Design review of the part built by this model. Coordinates are the model's own, in mm. Give positions to 0.01 mm unless a question says otherwise; leave off trailing zeros. Order: outer loops, then holes, each group sorted by start corner. A loop starts at its lowest first (then second) coordinate and runs counter-clockwise, first axis right, second up. Notation, with made-up numbers: M 78.25,-33.75 L 136.25,-33.75 A32 cw 136.25,5.25 Z; hole C 13.5,44.5 d2. An arc over 180 degrees is marked long. Answer as a JSON object with one key per item and string values.
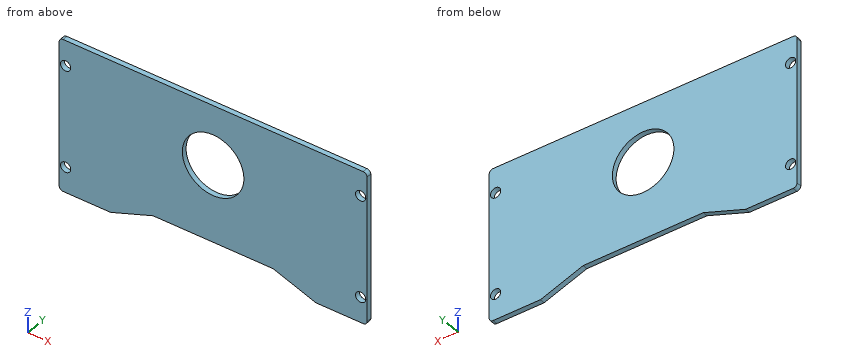
from build123d import *

# Parameters (mm, degrees)
SKETCH_1_W          = 120
SKETCH_1_H          = 60
EXTRUDE_1_DEPTH     = 2
SKETCH_2_R          = 2
CUT_EXTRUDE_1_DEPTH = 2
SKETCH_3_R          = 12
CUT_EXTRUDE_2_DEPTH = 2
FILLET_1_R          = 1.5


with BuildPart() as part:
    # 草图1 → 凸台-拉伸1 (new body)
    with BuildSketch(Plane(origin=(0, 0, 0), x_dir=(1, 0, 0), z_dir=(0, 1, 0))):
        with Locations((60, 30)):
            Rectangle(SKETCH_1_W, SKETCH_1_H)
    extrude(amount=EXTRUDE_1_DEPTH)

    # 草图2 → 切除-拉伸1 (cut)
    with BuildSketch(Plane(origin=(0, 2, 0), x_dir=(1, 0, 0), z_dir=(0, 1, 0))):
        with Locations(Location((117.5, 50, 0), (0, 0, 270))):
            Circle(SKETCH_2_R)
        with Locations(Location((117.5, 10, 0), (0, 0, 90))):
            Circle(SKETCH_2_R)
        with Locations(Location((2.5, 50, 0), (0, 0, 90))):
            Circle(SKETCH_2_R)
        with Locations(Location((2.5, 10, 0), (0, 0, 270))):
            Circle(SKETCH_2_R)
    extrude(amount=-CUT_EXTRUDE_1_DEPTH, mode=Mode.SUBTRACT)

    # 草图3 → 切除-拉伸2 (cut)
    with BuildSketch(Plane(origin=(0, 2, 0), x_dir=(1, 0, 0), z_dir=(0, 1, 0))):
        with Locations(Location((60, 23.556349186, 0), (0, 0, 270))):
            Circle(SKETCH_3_R)
        Polygon((20, 60), (36.582438817, 53.964485859), (83.417561183, 53.964485859), (100, 60), align=None)
    extrude(amount=-CUT_EXTRUDE_2_DEPTH, mode=Mode.SUBTRACT)

    # 圆角1
    fillet_1_edges = [part.edges().sort_by_distance(p)[0] for p in [
        (0, 1, -60),
        (120, 1, -60),
        (120, 1, 0),
        (0, 1, 0),
    ]]
    fillet(fillet_1_edges, radius=FILLET_1_R)


solid = part.part
(1) We need section B-B (x = 60). Write out the cut boundary in (y, z), plus the area to 3 significant figures.
Checked values:
{"outline": "M 0,-53.96 L 2,-53.96 L 2,-35.56 L 0,-35.56 Z; M 0,-11.56 L 2,-11.56 L 2,0 L 0,0 Z", "area": "59.9 mm^2"}
(2) We need section D-D (z = -25). Write out the cut boundary in (x, y).
Checked values:
{"outline": "M 0,0 L 48.09,0 L 48.09,2 L 0,2 Z; M 71.91,0 L 120,0 L 120,2 L 71.91,2 Z"}
(3) Insertion check: pin 1 (3 mm diameter, centred on x = 2.5, z = -50, fed in from -Y). The pin has a flat end and moves straight along its axis. Give the tip position at first contact, or say it passes through.
Checked values:
{"pin 1": "passes through"}
(4) We need section C-C (y = 1.55). Write out the cut boundary in (x, z).
Checked values:
{"outline": "M 0,-58.5 A1.5 ccw 1.5,-60 L 20,-60 L 36.58,-53.96 L 83.42,-53.96 L 100,-60 L 118.5,-60 A1.5 ccw 120,-58.5 L 120,-1.5 A1.5 ccw 118.5,0 L 1.5,0 A1.5 ccw 0,-1.5 Z; hole C 2.5,-50 d4; hole C 2.5,-10 d4; hole C 60,-23.56 d24; hole C 117.5,-50 d4; hole C 117.5,-10 d4"}
(5) To check wall thickness, follow L1, parallel to X at y = 0.9, z = -50; L2, parallel to X at y = 1.6, z = -8.5; L3, parallel to X at y = 0.6, z = -31.5. State the ranges of each line that lie inside material, in increasing order. Write a range as from..to.
Checked values:
{"L1": "x = 0..0.5, 4.5..115.5, 119.5..120", "L2": "x = 0..1.18, 3.82..116.18, 118.82..120", "L3": "x = 0..51.01, 68.99..120"}
(6) We need section A-A (z = -10). Write out the cut boundary in (x, y).
Checked values:
{"outline": "M 0,0 L 0.5,0 L 0.5,2 L 0,2 Z; M 4.5,0 L 115.5,0 L 115.5,2 L 4.5,2 Z; M 119.5,0 L 120,0 L 120,2 L 119.5,2 Z"}
